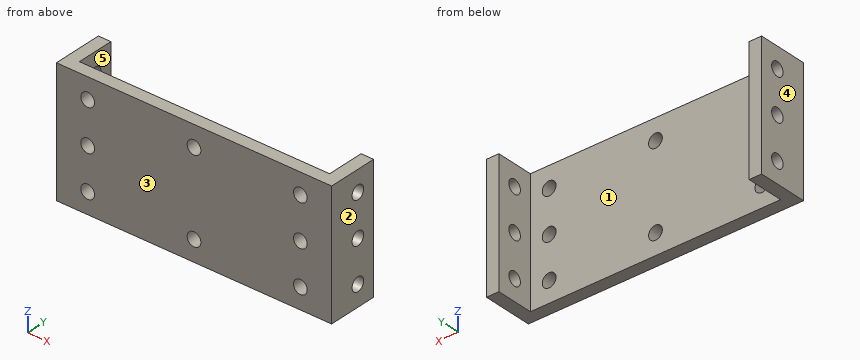
```python
from build123d import *

# Parameters (mm, degrees)
EXTRUDE_1_DEPTH     = 30
SKETCH_2_R          = 1.65
CUT_EXTRUDE_1_DEPTH = 74.054773971
CUT_EXTRUDE_2_REACH = 72.356
SKETCH_3_R          = 1.65
CUT_EXTRUDE_3_REACH = 72.356
SKETCH_4_R          = 1.65


with BuildPart() as part:
    # ｽｹｯﾁ1 → ﾎﾞｽ - 押し出し1 (new body)
    with BuildSketch(Plane.XY):
        Polygon((0, 0), (0, 9), (-3, 9), (-3, -3), (63, -3), (63, 9), (60, 9), (60, 0), align=None)
    extrude(amount=EXTRUDE_1_DEPTH)

    # ｽｹｯﾁ2 → ｶｯﾄ - 押し出し1 (cut, through all)
    with BuildSketch(Plane(origin=(63, 0, 0), x_dir=(0, 0, -1), z_dir=(1, 0, 0))):
        with Locations((-25, 4.5)):
            Circle(SKETCH_2_R)
        with Locations((-5, 4.5)):
            Circle(SKETCH_2_R)
        with Locations((-15, 4.5)):
            Circle(SKETCH_2_R)
    extrude(amount=-CUT_EXTRUDE_1_DEPTH, mode=Mode.SUBTRACT)

    # ｽｹｯﾁ3 → ｶｯﾄ - 押し出し2 (cut, up to next)
    with BuildSketch(Plane(origin=(0, 0, 0), x_dir=(1, 0, 0), z_dir=(0, 1, 0)), mode=Mode.PRIVATE) as cut_extrude_2_sk1:
        with Locations(Location((30, -5, 0), (0, 0, 180))):
            Circle(SKETCH_3_R)
    cut_extrude_2_tool1 = extrude(cut_extrude_2_sk1.sketch, amount=-CUT_EXTRUDE_2_REACH, mode=Mode.PRIVATE) & part.part
    # ｽｹｯﾁ3 → ｶｯﾄ - 押し出し2 (cut, up to next)
    with BuildSketch(Plane(origin=(0, 0, 0), x_dir=(1, 0, 0), z_dir=(0, 1, 0)), mode=Mode.PRIVATE) as cut_extrude_2_sk2:
        with Locations(Location((30, -25, 0), (0, 0, 180))):
            Circle(SKETCH_3_R)
    cut_extrude_2_tool2 = extrude(cut_extrude_2_sk2.sketch, amount=-CUT_EXTRUDE_2_REACH, mode=Mode.PRIVATE) & part.part
    add(cut_extrude_2_tool1.solids().sort_by_distance((30, 0, 5))[0], mode=Mode.SUBTRACT)
    add(cut_extrude_2_tool2.solids().sort_by_distance((30, 0, 25))[0], mode=Mode.SUBTRACT)

    # ｽｹｯﾁ4 → ｶｯﾄ - 押し出し3 (cut, up to next)
    with BuildSketch(Plane(origin=(0, 0, 0), x_dir=(1, 0, 0), z_dir=(0, 1, 0)), mode=Mode.PRIVATE) as cut_extrude_3_sk1:
        with Locations(Location((4.5, -5, 0), (0, 0, 180))):
            Circle(SKETCH_4_R)
    cut_extrude_3_tool1 = extrude(cut_extrude_3_sk1.sketch, amount=-CUT_EXTRUDE_3_REACH, mode=Mode.PRIVATE) & part.part
    # ｽｹｯﾁ4 → ｶｯﾄ - 押し出し3 (cut, up to next)
    with BuildSketch(Plane(origin=(0, 0, 0), x_dir=(1, 0, 0), z_dir=(0, 1, 0)), mode=Mode.PRIVATE) as cut_extrude_3_sk2:
        with Locations(Location((4.5, -15, 0), (0, 0, 180))):
            Circle(SKETCH_4_R)
    cut_extrude_3_tool2 = extrude(cut_extrude_3_sk2.sketch, amount=-CUT_EXTRUDE_3_REACH, mode=Mode.PRIVATE) & part.part
    # ｽｹｯﾁ4 → ｶｯﾄ - 押し出し3 (cut, up to next)
    with BuildSketch(Plane(origin=(0, 0, 0), x_dir=(1, 0, 0), z_dir=(0, 1, 0)), mode=Mode.PRIVATE) as cut_extrude_3_sk3:
        with Locations(Location((4.5, -25, 0), (0, 0, 180))):
            Circle(SKETCH_4_R)
    cut_extrude_3_tool3 = extrude(cut_extrude_3_sk3.sketch, amount=-CUT_EXTRUDE_3_REACH, mode=Mode.PRIVATE) & part.part
    # ｽｹｯﾁ4 → ｶｯﾄ - 押し出し3 (cut, up to next)
    with BuildSketch(Plane(origin=(0, 0, 0), x_dir=(1, 0, 0), z_dir=(0, 1, 0)), mode=Mode.PRIVATE) as cut_extrude_3_sk4:
        with Locations(Location((55.5, -25, 0), (0, 0, 180))):
            Circle(SKETCH_4_R)
    cut_extrude_3_tool4 = extrude(cut_extrude_3_sk4.sketch, amount=-CUT_EXTRUDE_3_REACH, mode=Mode.PRIVATE) & part.part
    # ｽｹｯﾁ4 → ｶｯﾄ - 押し出し3 (cut, up to next)
    with BuildSketch(Plane(origin=(0, 0, 0), x_dir=(1, 0, 0), z_dir=(0, 1, 0)), mode=Mode.PRIVATE) as cut_extrude_3_sk5:
        with Locations(Location((55.5, -15, 0), (0, 0, 180))):
            Circle(SKETCH_4_R)
    cut_extrude_3_tool5 = extrude(cut_extrude_3_sk5.sketch, amount=-CUT_EXTRUDE_3_REACH, mode=Mode.PRIVATE) & part.part
    # ｽｹｯﾁ4 → ｶｯﾄ - 押し出し3 (cut, up to next)
    with BuildSketch(Plane(origin=(0, 0, 0), x_dir=(1, 0, 0), z_dir=(0, 1, 0)), mode=Mode.PRIVATE) as cut_extrude_3_sk6:
        with Locations(Location((55.5, -5, 0), (0, 0, 180))):
            Circle(SKETCH_4_R)
    cut_extrude_3_tool6 = extrude(cut_extrude_3_sk6.sketch, amount=-CUT_EXTRUDE_3_REACH, mode=Mode.PRIVATE) & part.part
    add(cut_extrude_3_tool1.solids().sort_by_distance((4.5, 0, 5))[0], mode=Mode.SUBTRACT)
    add(cut_extrude_3_tool2.solids().sort_by_distance((4.5, 0, 15))[0], mode=Mode.SUBTRACT)
    add(cut_extrude_3_tool3.solids().sort_by_distance((4.5, 0, 25))[0], mode=Mode.SUBTRACT)
    add(cut_extrude_3_tool4.solids().sort_by_distance((55.5, 0, 25))[0], mode=Mode.SUBTRACT)
    add(cut_extrude_3_tool5.solids().sort_by_distance((55.5, 0, 15))[0], mode=Mode.SUBTRACT)
    add(cut_extrude_3_tool6.solids().sort_by_distance((55.5, 0, 5))[0], mode=Mode.SUBTRACT)


solid = part.part
```
Geometry check sheet. Reference: the model listing, model coordinates, mm. Face numbers are marked on the shaded views. A direction names the side the tool comes from. Give positions to 0.01 mm unless a question says otherwise; leave off trailing zeros. Order: outer loops, then holes, each group sorted by start corner. A loop starts at its lowest first (then second) coordinate and runs counter-clockwise, first axis right, second up. Notation, with made-up numbers: (35, -25.75) - (39, -25.75) arc R28 cw to (39, -7.75) - close; hole circle Ø5 at (-38.5, 40.25). An arc over 180 degrees is marked (long way). Answer in a Markdown table with one row per item. Add a question column.
Q1. Cross-section at D-D, the plane x = 30. Enter the section's corners in (y, z), then the cut area to 3 significant figures.
Q2. Tool access check on the marked faces 1 and 2. Record the directions out of +Z, -Z, +X, -X, +Y, -Y that give a thin tool (end or side, any length) a straight path to the whole face; none if there is none.
Q3. Cross-section at C-C, the plane y = 1.25. Enter the section's corners in (x, z), then the cut area to 3 significant figures.
Q4. Mould release check, pull along X, two halves, no side actions. Record for the marked faces 3, 4 and 5: pulls with the +X half, pulls with the -X half, needs draft (parallel to the pull), parting line crosses it, or undercut.
Q5. Material ranges on probe 1 along Z at (x, y) = (55.5, -2.3); probe 2 along X at (y, z) = (2.5, 22.5); probe 3 along Y at (x, z) = (61.8, 15), recorded low to high. Write a range as from..to.
Q6. Gauge pin test, flat ends, axial feed: pin 1 (2 mm diameter, centred on x = 6, z = 7, fed in from +Y); pin 2 (5.5 mm diameter, centred on x = 30, z = 5, fed in from -Y). Record the tip position at first contact, or that the pin passes through.
Q7. Cross-section at B-B, the plane z = 25. Enter the section's corners in (x, y).
Q8. Cross-section at A-A, the plane x = 4.5. Enter the section's corners in (y, z), then the cut area to 3 significant figures.
Check values:
| question | item | result |
|---|---|---|
| 1 | outline | (-3, 0) - (0, 0) - (0, 3.35) - (-3, 3.35) - close; (-3, 6.65) - (0, 6.65) - (0, 23.35) - (-3, 23.35) - close; (-3, 26.65) - (0, 26.65) - (0, 30) - (-3, 30) - close |
| 1 | area | 70.2 mm^2 |
| 2 | face 1 | +Z, -Z, +Y |
| 2 | face 2 | +Z, -Z, +X, +Y, -Y |
| 3 | outline | (-3, 0) - (0, 0) - (0, 30) - (-3, 30) - close; (60, 0) - (63, 0) - (63, 30) - (60, 30) - close |
| 3 | area | 180 mm^2 |
| 4 | face 3 | needs draft |
| 4 | face 4 | pulls with the -X half |
| 4 | face 5 | undercut |
| 5 | probe 1 | z = 0..3.35, 6.65..13.35, 16.65..23.35, 26.65..30 |
| 5 | probe 2 | x = -3..0, 60..63 |
| 5 | probe 3 | y = -3..2.85, 6.15..9 |
| 6 | pin 1 | stops at y = 0 |
| 6 | pin 2 | stops at y = -3 |
| 7 | outline | (-3, -3) - (2.85, -3) - (2.85, 0) - (0, 0) - (0, 2.85) - (-3, 2.85) - close; (-3, 6.15) - (0, 6.15) - (0, 9) - (-3, 9) - close; (6.15, -3) - (28.35, -3) - (28.35, 0) - (6.15, 0) - close; (31.65, -3) - (53.85, -3) - (53.85, 0) - (31.65, 0) - close; (57.15, -3) - (63, -3) - (63, 2.85) - (60, 2.85) - (60, 0) - (57.15, 0) - close; (60, 6.15) - (63, 6.15) - (63, 9) - (60, 9) - close |
| 8 | outline | (-3, 0) - (0, 0) - (0, 3.35) - (-3, 3.35) - close; (-3, 6.65) - (0, 6.65) - (0, 13.35) - (-3, 13.35) - close; (-3, 16.65) - (0, 16.65) - (0, 23.35) - (-3, 23.35) - close; (-3, 26.65) - (0, 26.65) - (0, 30) - (-3, 30) - close |
| 8 | area | 60.3 mm^2 |
